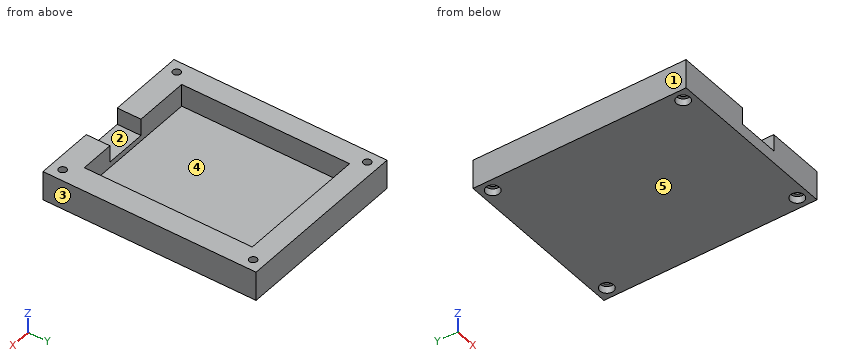
Autodesk Fusion 360 part; units mm, degrees
sketch "Sketch1" plane through (0, 0, 0) normal (0, 0, 1) x (1, 0, 0) in component "HackYeah (1)"
  line L0 (110, 210) -> (168, 210)
  line L1 (168, 210) -> (168, 135.669)
  line L2 (168, 135.669) -> (110, 135.669)
  line L3 (110, 135.669) -> (110, 210)
  line L4 (100.5, 219.5) -> (178.5, 219.5)
  line L5 (178.5, 219.5) -> (178.5, 125.169)
  line L6 (178.5, 125.169) -> (100.5, 125.169)
  line L7 (100.5, 125.169) -> (100.5, 219.5)
  circle A0 centre (105.5, 130.169) radius 1.7
  circle A1 centre (173.5, 130.169) radius 1.7
  circle A2 centre (105.5, 214.5) radius 1.7
  circle A3 centre (173.5, 214.5) radius 1.7
  circle A4 centre (105.5, 130.169) radius 3
  circle A5 centre (173.5, 130.169) radius 3
  circle A6 centre (105.5, 214.5) radius 3
  circle A7 centre (173.5, 214.5) radius 3
  dimension "d22" = 58
  dimension "d23" = 74.331
  dimension "d24" = 78
  dimension "d25" = 94.331
  dimension "d26" = 9.5
  dimension "d27" = 9.5
  dimension "d28" = 3.4
  dimension "d29" = 5
  dimension "d30" = 5
  dimension "d31" = 3.4
  dimension "d32" = 5
  dimension "d33" = 5
  dimension "d34" = 3.4
  dimension "d35" = 5
  dimension "d36" = 5
  dimension "d37" = 3.4
  dimension "d38" = 5
  dimension "d39" = 5
  dimension "d40" = 6
  dimension "d41" = 6
  dimension "d42" = 6
  dimension "d43" = 6
extrude "Extrude1" add sketch "Sketch1" along normal blind 9.9 from surface at 3.1 contours A4 | A5 | A6 | A7 makes body 1 at (102.7356, 213.3347, 9.7) makes body 2 at (108.2644, 131.3343, 9.7) makes body 3 at (171.4053, 212.3524, 9.7) makes body 4 at (176.2644, 131.3343, 9.7) in component "HackYeah (1)"
extrude "Extrude2" add sketch "Sketch1" along normal blind 13 contours L4 L5 L6 L7 bodies 1 2 3 4 in component "HackYeah (1)"
extrude "Extrude3" add sketch "Sketch1" along normal blind 3 contours L0 L1 L2 L3 bodies 1 in component "HackYeah (1)"
sketch "Sketch2" plane through (0, 0, 13) normal (0, 0, 1) x (-1, 0, 0) in component "HackYeah (1)"
  circle A0 centre (-105.5, -214.5) radius 1.7
  circle A1 centre (-173.5, -130.169) radius 1.7
  line L0 (-168, -135.669) -> (-110, -135.669)
  line L1 (-110, -135.669) -> (-110, -210)
  line L2 (-110, -210) -> (-168, -210)
  line L3 (-168, -210) -> (-168, -135.669)
  line L4 (-100.5, -125.169) -> (-178.5, -125.169)
  line L5 (-178.5, -125.169) -> (-178.5, -219.5)
  line L6 (-178.5, -219.5) -> (-100.5, -219.5)
  line L7 (-100.5, -219.5) -> (-100.5, -125.169)
  circle A2 centre (-105.5, -130.169) radius 1.7
  circle A3 centre (-173.5, -214.5) radius 1.7
  line L8 (24.854, 25.8508) -> (43.354, 25.8508)
  line L9 (43.354, 25.8508) -> (43.354, 16.3508)
  line L10 (43.354, 16.3508) -> (24.854, 16.3508)
  line L11 (24.854, 16.3508) -> (24.854, 25.8508)
  line L12 (-152.75, -125.169) -> (-134.25, -125.169)
  line L13 (-134.25, -125.169) -> (-134.25, -135.669)
  line L14 (-134.25, -135.669) -> (-152.75, -135.669)
  line L15 (-152.75, -135.669) -> (-152.75, -125.169)
  dimension "d51" = 18.5
  dimension "d52" = 9.5
  dimension "d53" = 18.5
  dimension "d54" = 10.5
  dimension "d55" = 25.75
extrude "Extrude4" cut sketch "Sketch2" against normal blind 7.5 contours L0 L4 L12 L13 L14 L15 bodies 1 in component "HackYeah (1)"
component "HackYeah (1)" placed x (1, 0, 0) y (0, 1, 0) z (0, 0, 1) at (0, 0, 0)
Here's how the part is built. I have some questions about the finished solid (model axes, mm). Face numbers are marked on the shaded views. A direction names the side the tool comes from. Coordinates: 2 decimals unless noted, no trailing zeros. Write each loop counter-clockwise with the first axis right and the second up, starting at its lowest first coordinate (ties: lowest second). Pieces come first, ordered by that corner, then holes. Notation, with made-up numbers: (-40, 6) - (-15, 6) arc R6 ccw to (-15, 16) - close; hole circle Ø4 at (11.5, 24.25). An arc over 180 degrees is marked (long way). Use one line per item in the form item = value.
1) Suppose I cut it at A-A, the plane x = 105.5. Write out the boundary of the cut face in (y, z).
Solved:
outline = (125.17, 0) - (127.17, 0) - (127.17, 3.1) - (128.47, 3.1) - (128.47, 13) - (125.17, 13) - close; (131.87, 3.1) - (133.17, 3.1) - (133.17, 0) - (211.5, 0) - (211.5, 3.1) - (212.8, 3.1) - (212.8, 13) - (131.87, 13) - close; (216.2, 3.1) - (217.5, 3.1) - (217.5, 0) - (219.5, 0) - (219.5, 13) - (216.2, 13) - close
2) Suppose I cut it at D-D, the plane z = 9.75. Write out the boundary of the cut face in (x, y).
Solved:
outline = (100.5, 125.17) - (134.25, 125.17) - (134.25, 135.67) - (110, 135.67) - (110, 210) - (168, 210) - (168, 135.67) - (152.75, 135.67) - (152.75, 125.17) - (178.5, 125.17) - (178.5, 219.5) - (100.5, 219.5) - close; hole circle Ø3.4 at (105.5, 130.17); hole circle Ø3.4 at (105.5, 214.5); hole circle Ø3.4 at (173.5, 130.17); hole circle Ø3.4 at (173.5, 214.5)
3) On a 3-axis mill with a long thin cutter (end or side, diameter ignored), from which of +Z, -Z, +X, -X, +Y, -Y can I reach the whole of each face in a straight line? I mean the marked faces 4 and 5. Say none if no direction works.
Solved:
face_4 = +Z
face_5 = -Z, +X, -X, +Y, -Y
4) Suppose I cut it at C-C, the plane y = 214.5. Write out the boundary of the cut face in (x, z).
Solved:
outline = (100.5, 0) - (102.5, 0) - (102.5, 3.1) - (103.8, 3.1) - (103.8, 13) - (100.5, 13) - close; (107.2, 3.1) - (108.5, 3.1) - (108.5, 0) - (170.5, 0) - (170.5, 3.1) - (171.8, 3.1) - (171.8, 13) - (107.2, 13) - close; (175.2, 3.1) - (176.5, 3.1) - (176.5, 0) - (178.5, 0) - (178.5, 13) - (175.2, 13) - close
5) Thinking about a two-plate mould opening in X: for the marked faces 1, 2 and 3, which applies, released by +X, released by -X, zero draft, split by the parting line, or undercut?
Solved:
face_1 = released by -X
face_2 = undercut
face_3 = released by +X
6) I need wall thicknesses on line 1 (Y direction, x = 173.5, z = 1); line 2 (Y direction, x = 105.5, z = 8.75); line 3 (X direction, y = 163.5, z = 11.25). Which ranges of each line are inside material? Lowest first, please.
Solved:
line_1 = 125.17 to 127.17, 133.17 to 211.5, 217.5 to 219.5
line_2 = 125.17 to 128.47, 131.87 to 212.8, 216.2 to 219.5
line_3 = 100.5 to 110, 168 to 178.5
7) Suppose I cut it at B-B, the plane y = 193.5. Write out the boundary of the cut face in (x, z), plus the area to 3 significant figures.
Solved:
outline = (100.5, 0) - (178.5, 0) - (178.5, 13) - (168, 13) - (168, 3) - (110, 3) - (110, 13) - (100.5, 13) - close
area = 434 mm2
8) I'm going to push flat-ended pins straight in: P1, Ø12, axis at x = 143.5, y = 190.5, coming from the +Z side; P2, Ø5.5, axis at x = 173.5, y = 130.169, coming from the +Z side; P3, Ø2, axis at x = 105.5, y = 130.169, coming from the -Z side; P4, Ø3.5, axis at x = 105.5, y = 214.5, coming from the -Z side. Where does each tip first touch, or does it pass through?
Solved:
P1 = 3
P2 = 13
P3 = through
P4 = 3.1
